Geometry: final body of the model. Coordinates: model frame, mm. Face numbers are marked on the shaded views. Round coordinates to 2 decimals unless told otherwise and drop trailing zeros. Loops run counter-clockwise (first coordinate to the right, second up) from the corner with the lowest first, then second, coordinate; pieces in that order, holes last. Notation, with made-up numbers: (-5, 63.25) - (26, 63.25) arc R12 ccw to (26, 71.25) - close; hole circle Ø2 at (19.5, 59). An arc over 180 degrees is marked (long way). Answer in a Markdown table with one row per item. Add a question column.
from build123d import *

# Parameters (mm, degrees)
SKETCH3_R           = 6
BOSS_EXTRUDE3_DEPTH = 12
SKETCH4_R           = 14
BOSS_EXTRUDE4_DEPTH = 8


with BuildPart() as part:
    # Sketch3 → Boss-Extrude3 (new body)
    with BuildSketch(Plane(origin=(0, 0, 0), x_dir=(1, 0, 0), z_dir=(0, 1, 0))):
        with BuildLine():
            ThreePointArc((-29.532846715, 2), (-28.947060278, 0.585786438), (-27.532846715, 0))
            Line((-27.532846715, 0), (36.467153285, 0))
            ThreePointArc((36.467153285, 0), (37.881366847, 0.585786438), (38.467153285, 2))
            Line((38.467153285, 2), (38.467153285, 42))
            ThreePointArc((38.467153285, 42), (20.082376974, 49.615223689), (12.467153285, 68))
            Line((12.467153285, 68), (-3.532846715, 68))
            ThreePointArc((-3.532846715, 68), (-11.148070404, 49.615223689), (-29.532846715, 42))
            Line((-29.532846715, 42), (-29.532846715, 2))
        make_face()
        with Locations(Location((-18.474270286, 17, 0), (0, 0, 270))):
            Circle(SKETCH3_R, mode=Mode.SUBTRACT)
        with Locations(Location((29.525729714, 17, 0), (0, 0, 270))):
            Circle(SKETCH3_R, mode=Mode.SUBTRACT)
    extrude(amount=-BOSS_EXTRUDE3_DEPTH)

    # Sketch4 → Boss-Extrude4 (add, symmetric)
    with BuildSketch(Plane(origin=(6.467153285, 0, 0), x_dir=(0, 0, -1), z_dir=(1, 0, 0))):
        with BuildLine():
            Line((17, 0), (83.047673955, 50.469532025))
            ThreePointArc((83.047673955, 50.469532025), (110.346676743, 51.747263432), (121.143218593, 26.641430746))
            Line((121.143218593, 26.641430746), (107, -12))
            Line((107, -12), (17, -12))
            Line((17, -12), (17, 0))
        make_face()
        with Locations((97.619641201, 31.399718953)):
            Circle(SKETCH4_R, mode=Mode.SUBTRACT)
    extrude(amount=BOSS_EXTRUDE4_DEPTH, both=True)


solid = part.part
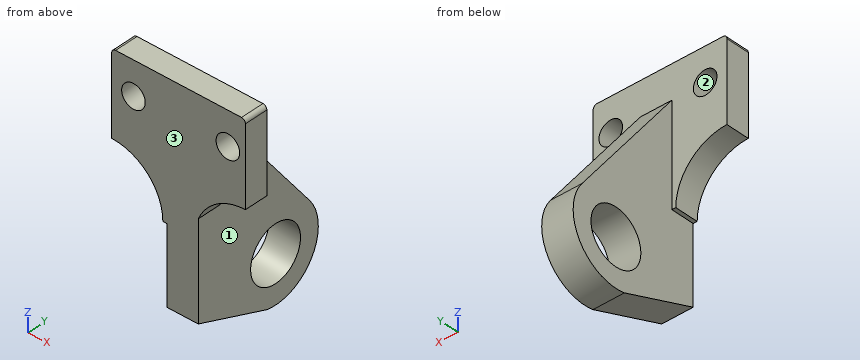
1) Section A-A, the plane z = -103.5. Return the cut outline in (x, y), and give its area (3 significant figures).
2) Material intervals for line 1 along X through (y, z) = (-6, -17); line 2 along X through (y, z) = (3.5, -97); line 3 along Y through (x, z) = (-21.5, -26.5), sorted ascending. Write a range as from..to.
3) Pull-direction query (X, two-part tool) for the marked faces 1, 2 and 3; classes: pulls with the +X half, pulls with the -X half, needs draft (parallel to the pull), parting line crosses it, or undercut.
4) Section D-D, the plane y = 6. Return the cut outline in (x, z), and give its area (3 significant figures).
5) Section B-B, the plane x = 33.5. Return the cut outline in (y, z), and give its area (3 significant figures).
6) Contact query for flat-ended pins moving along their axis: pin 1 Ø12 at (x, y) = (16, 20.5) entering from -Z; pin 2 Ø19 at (x, z) = (-18.47, -17) entering from -Y; pin 3 Ø22.5 at (y, z) = (31.4, -97.62) entering from +X; pin 4 Ø8 at (y, z) = (0, -101) entering from -X. Output: stop coordinate, or through.
7) Section C-C, the plane z = -47.5. Return the cut outline in (x, y), and give its area (3 significant figures).
Evaluation:
| question | item | result |
|---|---|---|
| 1 | outline | (-1.53, -12) - (14.47, -12) - (14.47, 18.69) - (-1.53, 18.69) - close; (-1.53, 44.1) - (14.47, 44.1) - (14.47, 54.67) - (-1.53, 54.67) - close |
| 1 | area | 660 mm² |
| 2 | line 1 | x = -29.53..-24.47, -12.47..23.53, 35.53..38.47 |
| 2 | line 2 | x = -1.53..14.47 |
| 2 | line 3 | y = -12..0 |
| 3 | face 1 | pulls with the +X half |
| 3 | face 2 | undercut |
| 3 | face 3 | needs draft |
| 4 | outline | (-1.53, -113.59) - (14.47, -113.59) - (14.47, -24.85) - (-1.53, -24.85) - close |
| 4 | area | 1,420 mm² |
| 5 | outline | (-12, -42.48) - (0, -42.48) - (0, -21.5) - (-12, -21.5) - close; (-12, -12.5) - (0, -12.5) - (0, 0) - (-12, 0) - close |
| 5 | area | 402 mm² |
| 6 | pin 1 | stops at z = -121.02 |
| 6 | pin 2 | stops at y = -12 |
| 6 | pin 3 | passes through |
| 6 | pin 4 | stops at x = -1.53 |
| 7 | outline | (-13.54, -12) - (22.47, -12) - (22.47, 0) - (14.47, 0) - (14.47, 23.31) - (-1.53, 23.31) - (-1.53, 0) - (-13.54, 0) - close |
| 7 | area | 805 mm² |
